Build history of the part. All positions in model axes, mm. Face numbers are marked on the shaded views. Give positions to 0.01 mm unless a question says otherwise; leave off trailing zeros. Order: outer loops, then holes, each group sorted by start corner. A loop starts at its lowest first (then second) coordinate and runs counter-clockwise, first axis right, second up. Notation, with made-up numbers: M -9,73.25 L 24,73.25 A15 ccw 24,79.25 Z; hole C 55,30 d11. An arc over 180 degrees is marked long. Use CSV: the item, a comma, the result in double quotes. Start each with the question number.
Item 1: Band-saw the part on B-B on x = -36. Write the cut outline in (y, z).
Item 2: Band-saw the part on C-C on z = -50. Write the cut outline in (x, y), plus the area to 3 significant figures.
Item 3: Pin check, flat tips, straight feed: P1, Ø3, axis at y = -4.5, z = -36.5, coming from the -X side; P2, Ø5.5, axis at x = -26.5, y = -5, coming from the -Z side; P3, Ø2, axis at x = -43.5, y = -2, coming from the +Z side; P4, Ø8, axis at y = -5, z = -32.5, coming from the +X side. Stop position of each tip, or through.
Item 4: Band-saw the part on A-A on y = -5. Write the cut outline in (x, z).
Item 5: Two-plate mould, pull along X, no slides. Class the marked faces 1, 2 and 3: pulls with the +X half, pulls with the -X half, needs draft (parallel to the pull), parting line crosses it, or undercut.
Item 6: Wall check: line 1 along X through (y, z) = (3.5, -14.5); line 2 along X through (y, z) = (-6.75, -23); line 3 along Y through (x, z) = (-10.5, -2.5). Give the ranges that are in metal, low to high.
Autodesk Inventor part; units mm, degrees
ref_plane "YZ Plane" through (0, 0, 0) normal (1, 0, 0) x (0, 1, 0)
ref_plane "XZ Plane" through (0, 0, 0) normal (0, 1, 0) x (-1, 0, 0)
ref_plane "XY Plane" through (0, 0, 0) normal (0, 0, 1) x (1, 0, 0)
sketch "스케치1" plane through (0, 0, 0) normal (0, 1, 0) x (-1, 0, 0)
  line L0 (0, 0) -> (64.8, 0)
  line L1 (64.8, 0) -> (64.8, -64.8)
  line L2 (64.8, -64.8) -> (0, -64.8)
  line L3 (0, -64.8) -> (0, 0)
  dimension "d0" = 64.8
  dimension "d1" = 64.8
extrude "돌출1" add sketch "스케치1" along normal blind 5
sketch "스케치2" plane through (0, 5, 0) normal (0, 1, 0) x (1, 0, 0)
  line L0 (-2.4, 2.4) -> (-62.4, 2.4)
  line L1 (-62.4, 2.4) -> (-62.4, 62.4)
  line L2 (-62.4, 62.4) -> (-2.4, 62.4)
  line L3 (-2.4, 62.4) -> (-2.4, 2.4)
  line L4 (-64.8, 0) -> (0, 0)
  line L5 (0, 0) -> (0, 64.8)
  line L6 (-64, 0.8) -> (-0.8, 0.8)
  line L7 (-0.8, 0.8) -> (-0.8, 64)
  line L8 (-0.8, 64) -> (-64, 64)
  line L9 (-64, 64) -> (-64, 0.8)
  line L10 (0, 64.8) -> (-64.8, 64.8)
  dimension "d54" = 60
  dimension "d55" = 1.6
  dimension "d56" = 1.6
  dimension "d57" = 1.6
  dimension "d58" = 1.6
  dimension "d59" = 2.4
  dimension "d60" = 2.4
  dimension "d61" = 2.4
extrude "돌출2" cut sketch "스케치2" against normal blind 1.6
sketch "스케치7" plane through (0, 0, 0) normal (0, -1, 0) x (1, 0, 0)
  line L0 (-29.9, -22.4) -> (-24.9, -22.4)
  line L1 (-24.9, -22.4) -> (-24.9, -42.4)
  line L2 (-24.9, -42.4) -> (-29.9, -42.4)
  line L3 (-29.9, -42.4) -> (-29.9, -22.4)
  line L4 (-39.9, -22.4) -> (-34.9, -22.4)
  line L5 (-34.9, -22.4) -> (-34.9, -42.4)
  line L6 (-34.9, -42.4) -> (-39.9, -42.4)
  line L7 (-39.9, -42.4) -> (-39.9, -22.4)
  line L8 (0, 0) -> (0, -64.8)
  line L9 (-34.9, -42.4) -> (-29.9, -42.4)
  line L10 (-64.8, 0) -> (0, 0)
  point P0 (0, -32.4)
  point P1 (-24.9, -32.4)
  point P2 (-32.4, -42.4)
  point P3 (-32.4, 0)
  dimension "d37" = 5
  dimension "d38" = 20
  dimension "d41" = 10
extrude "돌출7" add sketch "스케치7" along normal blind 10
sketch "스케치8" plane through (-24.9, 0, -22.4) normal (1, 0, 0) x (0, 0, -1)
  circle A0 centre (6.0516, -5) radius 1.25
  circle A1 centre (13.9484, -5) radius 1.25
  line L0 (13.9484, -5) -> (6.0516, -5)
  line L1 (-22.4, 0) -> (42.4, 0)
  line L2 (0, 0) -> (0, -10)
  point P0 (10, -5)
  point P1 (10, 0)
  point P2 (0, -5)
  dimension "d48" = 2.5
  dimension "d49" = 2.5
extrude "돌출8" cut sketch "스케치8" against normal blind 15
properties part number "사각형 OV-PAM 5패턴 상단"
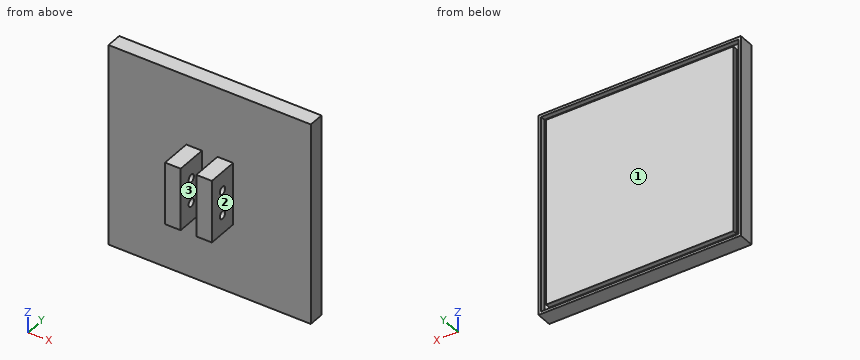
Model answer:
1,outline,"M -10,-42.4 L 0,-42.4 L 0,-64.8 L 5,-64.8 L 5,-64 L 3.4,-64 L 3.4,-62.4 L 5,-62.4 L 5,-2.4 L 3.4,-2.4 L 3.4,-0.8 L 5,-0.8 L 5,0 L 0,0 L 0,-22.4 L -10,-22.4 Z; hole C -5,-36.35 d2.5; hole C -5,-28.45 d2.5"
2,outline,"M -64.8,0 L 0,0 L 0,5 L -0.8,5 L -0.8,3.4 L -2.4,3.4 L -2.4,5 L -62.4,5 L -62.4,3.4 L -64,3.4 L -64,5 L -64.8,5 Z"
2,area,"319 mm^2"
3,P1,"stops at x = -39.9"
3,P2,"stops at z = -42.4"
3,P3,"passes through"
3,P4,"stops at x = -24.9"
4,outline,"M -39.9,-42.4 L -34.9,-42.4 L -34.9,-37.6 L -39.9,-37.6 Z; M -39.9,-35.1 L -34.9,-35.1 L -34.9,-29.7 L -39.9,-29.7 Z; M -39.9,-27.2 L -34.9,-27.2 L -34.9,-22.4 L -39.9,-22.4 Z; M -29.9,-42.4 L -24.9,-42.4 L -24.9,-37.6 L -29.9,-37.6 Z; M -29.9,-35.1 L -24.9,-35.1 L -24.9,-29.7 L -29.9,-29.7 Z; M -29.9,-27.2 L -24.9,-27.2 L -24.9,-22.4 L -29.9,-22.4 Z"
5,face 1,"needs draft"
5,face 2,"pulls with the +X half"
5,face 3,"undercut"
6,line 1,"x = -64.8 to -64, -62.4 to -2.4, -0.8 to 0"
6,line 2,"x = -39.9 to -34.9, -29.9 to -24.9"
6,line 3,"y = 0 to 5"
